Can you work these out from the model? Positions are in its coordinate system, mm. Face numbers are marked on the shaded views. A direction names the side the tool comes from. Give positions to 0.01 mm unless a question says otherwise; leave off trailing zeros. Loops run counter-clockwise (first coordinate to the right, second up) from the corner with the lowest first, then second, coordinate; pieces in that order, holes last. Notation, with made-up numbers: (25.5, -5.5) -> (34.5, -5.5) arc R20 ccw to (34.5, 28.5) -> close; hole circle Ø4 at (-8.5, 35.25). An arc over 180 degrees is marked (long way). Return JSON: item names as keys, results as strings. Group by question number.
Q1. Suppose I cut it at C-C, the plane z = -26.75. Please give me the cut outline in (x, y) (3 decimals).
Q2. Suppose I cut it at B-B, the plane x = -11. Please give me the cut outline in (y, z), and give its area (3 significant figures).
Q3. Suppose I cut it at A-A, the plane z = -47.5. Please give me the cut outline in (x, y), and give its area (3 significant figures).
Q4. Will these pins go through, and if not, where does the flat tip stop? pin 1 (6 mm diameter, centred on y = 9.5, z = -39, fed in from -X); pin 2 (3 mm diameter, centred on y = -14, z = -76.5, fed in from +X) (3 decimals); pin 3 (10 mm diameter, centred on x = -9, y = 24.5, fed in from +Z); pin 4 (2 mm diameter, centred on x = 17, z = -49, fed in from +Y).
Q5. Which directions (+Z, -Z, +X, -X, +Y, -Y) give clear straight access to the entire face, cutting with the end or side of a thin tool? Please do the marked faces 1, 2 and 3.
Q6. I need wall thicknesses on line 1 along Y through (x, z) = (-10, -5.65); line 2 along Y through (x, z) = (10, -3.35); line 3 along X through (y, z) = (25, -2). Which ranges of each line are inside material? Lowest first, please. Write a range as [from, to].
```python
from build123d import *

# Parameters (mm, degrees)
SKETCH2_W            = 40
SKETCH2_H            = 65.4
SKETCH2_R            = 2.5
BOSS_EXTRUDE1_DEPTH  = 6
SKETCH3_W            = 4.5
SKETCH3_H            = 40
BOSS_EXTRUDE2_DEPTH  = 52
CUT_EXTRUDE1_REACH   = 6.5
SKETCH4_R            = 12.573151632
SKETCH4_R_2          = 1.5
SKETCH5_R            = 4.5
CUT_EXTRUDE2_DEPTH   = 1.5
SKETCH6_R            = 3
CUT_EXTRUDE3_DEPTH   = 2.5
FILLET1_R            = 5
SKETCH11_R           = 2.5
BOSS_EXTRUDE6_DEPTH  = 4.5
FILLET2_R            = 3
SKETCH9_R            = 3.175
BOSS_EXTRUDE15_DEPTH = 4.5
SKETCH24_R           = 3.175
CUT_EXTRUDE11_DEPTH  = 4.5
SKETCH15_R           = 3
CUT_EXTRUDE12_DEPTH  = 2.5
SKETCH25_W           = 40
SKETCH25_H           = 9
BOSS_EXTRUDE16_DEPTH = 52.75
SKETCH28_W           = 40
SKETCH28_H           = 2
CUT_EXTRUDE15_DEPTH  = 3
SKETCH33_W           = 40
SKETCH33_H           = 5
CUT_EXTRUDE18_DEPTH  = 3
FILLET7_R            = 1
FILLET8_R            = 5
SKETCH31_W           = 40
SKETCH31_H           = 9.0424
CUT_EXTRUDE16_DEPTH  = 6
SKETCH32_R           = 2
CUT_EXTRUDE17_DEPTH  = 4
SKETCH34_R           = 2.5
CUT_EXTRUDE19_DEPTH  = 9
CUT_EXTRUDE20_DEPTH  = 10
FILLET9_R            = 5


with BuildPart() as part:
    # Sketch2 → Boss-Extrude1 (new body)
    with BuildSketch(Plane.XY):
        with Locations((0, 12.7)):
            Rectangle(SKETCH2_W, SKETCH2_H)
        with Locations((0, 35.4)):
            Circle(SKETCH2_R, mode=Mode.SUBTRACT)
        with Locations((0, 15.4)):
            Circle(SKETCH2_R, mode=Mode.SUBTRACT)
        with Locations((-10, 25.4)):
            Circle(SKETCH2_R, mode=Mode.SUBTRACT)
        with Locations((10, 25.4)):
            Circle(SKETCH2_R, mode=Mode.SUBTRACT)
    extrude(amount=-BOSS_EXTRUDE1_DEPTH)

    # Sketch3 → Boss-Extrude2 (add)
    with BuildSketch(Plane(origin=(0, 0, -6), x_dir=(-1, 0, 0), z_dir=(0, 0, -1))):
        with Locations((-17.75, 0)):
            Rectangle(SKETCH3_W, SKETCH3_H)
    extrude(amount=BOSS_EXTRUDE2_DEPTH)

    # Sketch4 → Cut-Extrude1 (cut, up to next)
    with BuildSketch(Plane.ZY.offset(-15.5), mode=Mode.PRIVATE) as cut_extrude1_sk1:
        with Locations((-32, 0)):
            Circle(SKETCH4_R)
    cut_extrude1_tool1 = extrude(cut_extrude1_sk1.sketch, amount=-CUT_EXTRUDE1_REACH, mode=Mode.PRIVATE) & part.part
    add(cut_extrude1_tool1.solids().sort_by_distance((15.5, 0, -32))[0], mode=Mode.SUBTRACT)
    # Sketch4 → Cut-Extrude1 (cut, up to next)
    with BuildSketch(Plane.ZY.offset(-15.5), mode=Mode.PRIVATE) as cut_extrude1_sk2:
        with Locations((-16.5, 15.5)):
            Circle(SKETCH4_R_2)
    cut_extrude1_tool2 = extrude(cut_extrude1_sk2.sketch, amount=-CUT_EXTRUDE1_REACH, mode=Mode.PRIVATE) & part.part
    add(cut_extrude1_tool2.solids().sort_by_distance((15.5, 15.5, -16.5))[0], mode=Mode.SUBTRACT)
    # Sketch4 → Cut-Extrude1 (cut, up to next)
    with BuildSketch(Plane.ZY.offset(-15.5), mode=Mode.PRIVATE) as cut_extrude1_sk3:
        with Locations((-16.5, -15.5)):
            Circle(SKETCH4_R_2)
    cut_extrude1_tool3 = extrude(cut_extrude1_sk3.sketch, amount=-CUT_EXTRUDE1_REACH, mode=Mode.PRIVATE) & part.part
    add(cut_extrude1_tool3.solids().sort_by_distance((15.5, -15.5, -16.5))[0], mode=Mode.SUBTRACT)
    # Sketch4 → Cut-Extrude1 (cut, up to next)
    with BuildSketch(Plane.ZY.offset(-15.5), mode=Mode.PRIVATE) as cut_extrude1_sk4:
        with Locations((-47.5, -15.5)):
            Circle(SKETCH4_R_2)
    cut_extrude1_tool4 = extrude(cut_extrude1_sk4.sketch, amount=-CUT_EXTRUDE1_REACH, mode=Mode.PRIVATE) & part.part
    add(cut_extrude1_tool4.solids().sort_by_distance((15.5, -15.5, -47.5))[0], mode=Mode.SUBTRACT)
    # Sketch4 → Cut-Extrude1 (cut, up to next)
    with BuildSketch(Plane.ZY.offset(-15.5), mode=Mode.PRIVATE) as cut_extrude1_sk5:
        with Locations((-47.5, 15.5)):
            Circle(SKETCH4_R_2)
    cut_extrude1_tool5 = extrude(cut_extrude1_sk5.sketch, amount=-CUT_EXTRUDE1_REACH, mode=Mode.PRIVATE) & part.part
    add(cut_extrude1_tool5.solids().sort_by_distance((15.5, 15.5, -47.5))[0], mode=Mode.SUBTRACT)

    # Sketch5 → Cut-Extrude2 (cut)
    with BuildSketch(Plane(origin=(0, 0, -6), x_dir=(-1, 0, 0), z_dir=(0, 0, -1))):
        with Locations((0, 35.4)):
            Circle(SKETCH5_R)
        with Locations((10, 25.4)):
            Circle(SKETCH5_R)
        with Locations((0, 15.4)):
            Circle(SKETCH5_R)
        with Locations((-10, 25.4)):
            Circle(SKETCH5_R)
    extrude(amount=-CUT_EXTRUDE2_DEPTH, mode=Mode.SUBTRACT)

    # Sketch6 → Cut-Extrude3 (cut)
    with BuildSketch(Plane.ZY.offset(-15.5)):
        with Locations((-16.5, 15.5)):
            Circle(SKETCH6_R)
        with Locations((-47.5, 15.5)):
            Circle(SKETCH6_R)
        with Locations((-47.5, -15.5)):
            Circle(SKETCH6_R)
        with Locations((-16.5, -15.5)):
            Circle(SKETCH6_R)
    extrude(amount=-CUT_EXTRUDE3_DEPTH, mode=Mode.SUBTRACT)

    # Fillet1
    fillet1_edges = [part.edges().sort_by_distance(p)[0] for p in [
        (-20, -20, -3),
    ]]
    fillet(fillet1_edges, radius=FILLET1_R)

    # Sketch11 → Boss-Extrude6 (add)
    with BuildSketch(Plane.ZY.offset(-15.5)):
        with BuildLine():
            Line((-58, -19.943670675), (-58, 19.943670675))
            ThreePointArc((-58, 19.943670675), (-64.026515977, 18.5297479), (-69.332027993, 15.34076457))
            ThreePointArc((-69.332027993, 15.34076457), (-72.76360296, 11.640241353), (-75.159610133, 7.198538025))
            ThreePointArc((-75.159610133, 7.198538025), (-76.5, 0), (-75.159610133, -7.198538025))
            ThreePointArc((-75.159610133, -7.198538025), (-72.76360296, -11.640241353), (-69.332027993, -15.34076457))
            ThreePointArc((-69.332027993, -15.34076457), (-64.026515977, -18.5297479), (-58, -19.943670675))
        make_face()
        with BuildLine():
            ThreePointArc((-75.159610133, 7.198538025), (-72.76360296, 11.640241353), (-69.332027993, 15.34076457))
            Line((-69.332027993, 15.34076457), (-73.799349609, 18.20790773))
            ThreePointArc((-73.799349609, 18.20790773), (-80.70790773, 16.700650391), (-79.200650391, 9.79209227))
            Line((-79.200650391, 9.79209227), (-75.159610133, 7.198538025))
        make_face()
        with Locations((-76.5, 14)):
            Circle(SKETCH11_R, mode=Mode.SUBTRACT)
        with BuildLine():
            Line((-73.799349609, -18.20790773), (-69.332027993, -15.34076457))
            ThreePointArc((-69.332027993, -15.34076457), (-72.76360296, -11.640241353), (-75.159610133, -7.198538025))
            Line((-75.159610133, -7.198538025), (-79.200650391, -9.79209227))
            ThreePointArc((-79.200650391, -9.79209227), (-80.70790773, -16.700650391), (-73.799349609, -18.20790773))
        make_face()
        with Locations((-76.5, -14)):
            Circle(SKETCH11_R, mode=Mode.SUBTRACT)
    extrude(amount=-BOSS_EXTRUDE6_DEPTH)

    # Fillet2
    fillet2_edges = [part.edges().sort_by_distance(p)[0] for p in [
        (17.75, -15.34076457, -69.332027993),
        (17.75, -7.198538025, -75.159610133),
        (17.75, 7.198538025, -75.159610133),
        (17.75, 15.34076457, -69.332027993),
    ]]
    fillet(fillet2_edges, radius=FILLET2_R)

    # Sketch9 → Boss-Extrude15 (add)
    with BuildSketch(Plane.ZY.offset(-15.5)):
        with BuildLine():
            Line((-32.75, -22), (-32.75, -18.434411342))
            Line((-32.75, -18.434411342), (-20.75, -18.434411342))
            Line((-20.75, -18.434411342), (-20.75, -22))
            ThreePointArc((-20.75, -22), (-26.75, -28), (-32.75, -22))
        make_face()
        with Locations((-26.75, -22)):
            Circle(SKETCH9_R, mode=Mode.SUBTRACT)
        with BuildLine():
            Line((-24.75, 21), (-24.75, 17.603718698))
            Line((-24.75, 17.603718698), (-12.75, 17.603718698))
            Line((-12.75, 17.603718698), (-12.75, 21))
            ThreePointArc((-12.75, 21), (-18.75, 27), (-24.75, 21))
        make_face()
        with Locations((-18.75, 21)):
            Circle(SKETCH9_R, mode=Mode.SUBTRACT)
    extrude(amount=-BOSS_EXTRUDE15_DEPTH)

    # Sketch24 → Cut-Extrude11 (cut)
    with BuildSketch(Plane.ZY.offset(-15.5)):
        with Locations((-18.75, 21)):
            Circle(SKETCH24_R)
        with Locations((-26.75, -22)):
            Circle(SKETCH24_R)
    extrude(amount=-CUT_EXTRUDE11_DEPTH, mode=Mode.SUBTRACT)

    # Sketch15 → Cut-Extrude12 (cut)
    with BuildSketch(Plane.ZY.offset(-15.5)):
        with Locations((-16.5, 15.5)):
            Circle(SKETCH15_R)
    extrude(amount=-CUT_EXTRUDE12_DEPTH, mode=Mode.SUBTRACT)

    # Sketch25 → Boss-Extrude16 (add)
    with BuildSketch(Plane(origin=(0, 45.4, 0), x_dir=(1, 0, 0), z_dir=(0, 1, 0))):
        with Locations((0, 1.5)):
            Rectangle(SKETCH25_W, SKETCH25_H)
    extrude(amount=BOSS_EXTRUDE16_DEPTH)

    # Sketch28 → Cut-Extrude15 (cut)
    with BuildSketch(Plane.XY.offset(3)):
        with Locations((0, 46.4)):
            Rectangle(SKETCH28_W, SKETCH28_H)
    extrude(amount=-CUT_EXTRUDE15_DEPTH, mode=Mode.SUBTRACT)

    # Sketch33 → Cut-Extrude18 (cut)
    with BuildSketch(Plane.XY.offset(3)):
        with Locations((0, 49.9)):
            Rectangle(SKETCH33_W, SKETCH33_H)
    extrude(amount=-CUT_EXTRUDE18_DEPTH, mode=Mode.SUBTRACT)

    # Fillet7
    fillet7_edges = [part.edges().sort_by_distance(p)[0] for p in [
        (0, 52.4, 3),
        (0, 52.4, 0),
    ]]
    fillet(fillet7_edges, radius=FILLET7_R)

    # Fillet8
    fillet8_edges = [part.edges().sort_by_distance(p)[0] for p in [
        (20, 98.15, -1.5),
        (-20, 98.15, -1.5),
    ]]
    fillet(fillet8_edges, radius=FILLET8_R)

    # Sketch31 → Cut-Extrude16 (cut)
    with BuildSketch(Plane(origin=(0, 0, -6), x_dir=(-1, 0, 0), z_dir=(0, 0, -1))):
        with Locations((0, 65.9212)):
            Rectangle(SKETCH31_W, SKETCH31_H)
        with Locations((0, 79.3136)):
            Rectangle(SKETCH31_W, SKETCH31_H)
    extrude(amount=-CUT_EXTRUDE16_DEPTH, mode=Mode.SUBTRACT)

    # Sketch32 → Cut-Extrude17 (cut, through all)
    with BuildSketch(Plane(origin=(0, 0, 0), x_dir=(-1, 0, 0), z_dir=(0, 0, -1))):
        with Locations((0, 79.3136)):
            Circle(SKETCH32_R)
        with Locations((0, 65.9212)):
            Circle(SKETCH32_R)
    extrude(amount=-CUT_EXTRUDE17_DEPTH, mode=Mode.SUBTRACT)

    # Sketch34 → Cut-Extrude19 (cut)
    with BuildSketch(Plane(origin=(0, 0, -6), x_dir=(-1, 0, 0), z_dir=(0, 0, -1))):
        with Locations((0, 90.9924)):
            Circle(SKETCH34_R)
    extrude(amount=-CUT_EXTRUDE19_DEPTH, mode=Mode.SUBTRACT)

    # Sketch35 → Cut-Extrude20 (cut)
    with BuildSketch(Plane(origin=(0, 0, -6), x_dir=(-1, 0, 0), z_dir=(0, 0, -1))):
        Polygon((-0.25, -20), (0, 0), (20, 0), (20, -20), align=None)
    extrude(amount=-CUT_EXTRUDE20_DEPTH, mode=Mode.SUBTRACT)

    # Fillet9
    fillet9_edges = [part.edges().sort_by_distance(p)[0] for p in [
        (0.25, -20, -3),
        (0, 0, -3),
        (-20, 0, -3),
    ]]
    fillet(fillet9_edges, radius=FILLET9_R)


solid = part.part
```
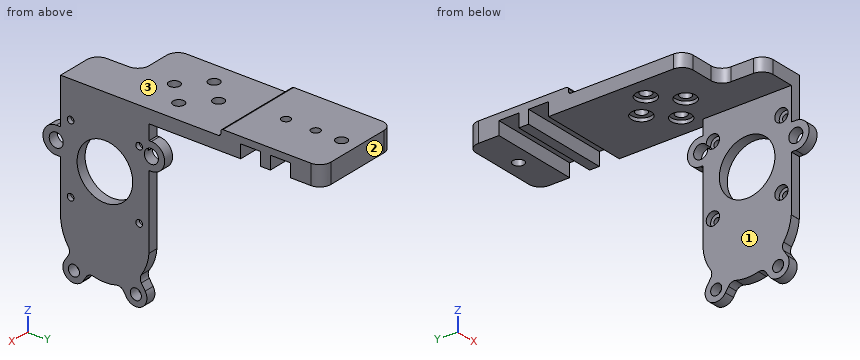
Ans:
{
 "1": {"outline": "(15.5, -28) -> (20, -28) -> (20, -25.175) -> (15.5, -25.175) -> close; (15.5, -18.825) -> (20, -18.825) -> (20, -11.425) -> (15.5, -11.425) -> close; (15.5, 11.425) -> (20, 11.425) -> (20, 20) -> (15.5, 20) -> close"},
 "2": {"outline": "(0, -6) -> (21.01, -6) -> (21.01, -4.5) -> (23.11, -4.5) -> (23.11, 0) -> (0, 0) -> close; (27.69, -4.5) -> (29.79, -4.5) -> (29.79, -6) -> (61.4, -6) -> (61.4, 0) -> (70.44, 0) -> (70.44, -6) -> (74.79, -6) -> (74.79, 0) -> (83.83, 0) -> (83.83, -6) -> (98.15, -6) -> (98.15, 3) -> (53.4, 3) arc R1 ccw to (52.4, 2) -> (52.4, 1) arc R1 cw to (51.4, 0) -> (27.69, 0) -> close", "area": "584 mm^2"},
 "3": {"outline": "(15.5, -20) -> (20, -20) -> (20, -17) -> (18, -17) -> (18, -18.5) -> (15.5, -18.5) -> close; (15.5, -12.5) -> (18, -12.5) -> (18, -14) -> (20, -14) -> (20, 14) -> (18, 14) -> (18, 12.5) -> (15.5, 12.5) -> close; (15.5, 18.5) -> (18, 18.5) -> (18, 17) -> (20, 17) -> (20, 20) -> (15.5, 20) -> close", "area": "138 mm^2"},
 "4": {"pin 1": "stops at x = 15.5", "pin 2": "passes through", "pin 3": "stops at z = 0", "pin 4": "stops at y = 20"},
 "5": {"face 1": "-Z, -X, +Y, -Y", "face 2": "+Z, -Z, +X, -X, +Y", "face 3": "+Z, +X, -X, -Y"},
 "6": {"line 1": "y = [0, 20.9], [29.9, 61.4], [70.44, 74.79], [83.83, 98.15]", "line 2": "y = [-20, 22.9], [27.9, 61.4], [70.44, 74.79], [83.83, 98.15]", "line 3": "x = [-20, -12.47], [-7.53, 7.53], [12.47, 20]"}
}
